from build123d import *

# Parameters (mm, degrees)
CROQUIS1_W              = 80
CROQUIS1_H              = 80
SALIENTE_EXTRUIR2_DEPTH = 2.7
CROQUIS2_R              = 2.5
CORTAR_EXTRUIR1_DEPTH   = 2.7
CROQUIS4_R              = 7.5
CORTAR_EXTRUIR2_DEPTH   = 2.7


with BuildPart() as part:
    # Croquis1 → Saliente-Extruir2 (new body)
    with BuildSketch(Plane.XY):
        with Locations((-42.7, 0)):
            Rectangle(CROQUIS1_W, CROQUIS1_H)
    extrude(amount=-SALIENTE_EXTRUIR2_DEPTH)

    # Croquis2 → Cortar-Extruir1 (cut)
    with BuildSketch(Plane(origin=(0, 0, -2.7), x_dir=(-1, 0, 0), z_dir=(0, 0, -1))):
        with Locations((67.7, 0)):
            Circle(CROQUIS2_R)
        with Locations((42.7, 0)):
            Circle(CROQUIS2_R)
    extrude(amount=-CORTAR_EXTRUIR1_DEPTH, mode=Mode.SUBTRACT)

    # Croquis4 → Cortar-Extruir2 (cut)
    with BuildSketch(Plane(origin=(0, 0, -2.7), x_dir=(-1, 0, 0), z_dir=(0, 0, -1))):
        with Locations((22.7, 23.2)):
            Circle(CROQUIS4_R)
    extrude(amount=-CORTAR_EXTRUIR2_DEPTH, mode=Mode.SUBTRACT)


solid = part.part
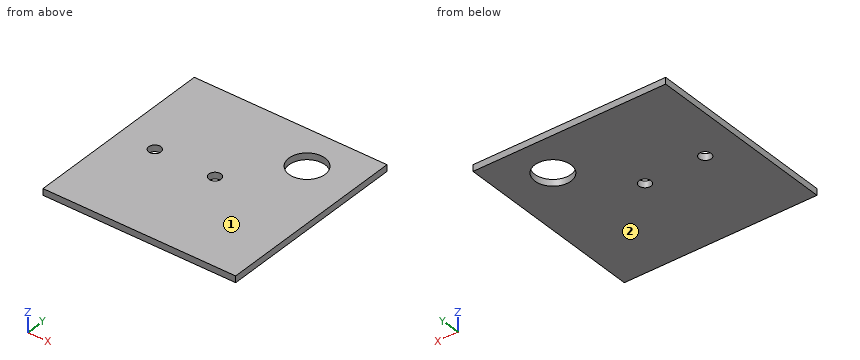
For this review, take the finished solid that the model builds, in its own axes (mm). Face numbers are marked on the shaded views. Coordinates: 2 decimals unless noted, no trailing zeros. Write each loop counter-clockwise with the first axis right and the second up, starting at its lowest first coordinate (ties: lowest second). Pieces come first, ordered by that corner, then holes. Notation, with made-up numbers: (18.5, 15.5) -> (67.5, 15.5) arc R15 ccw to (67.5, 25.5) -> close; hole circle Ø2 at (44, 46). An arc over 180 degrees is marked (long way). Write each question's results on one line, items separated by ' | '. Start each with the question number.
1) Wall thickness on L1, parallel to Y at x = -22.7, z = -2.05; L2, parallel to X at y = 1.5, z = -1.85; L3, parallel to Y at x = -67.7, z = -1.4: over which ranges is each line inside the solid? List them lowest first. Write a range as [from, to].
2) Consider section A-A (x = -67.7). Write out the cut boundary in (y, z), plus the area to 4 significant figures.
3) Consider section B-B (y = 23.2). Write out the cut boundary in (x, z), plus the area to 4 significant figures.
4) Consider section D-D (z = -2.05). Write out the cut boundary in (x, y), plus the area to 3 significant figures.
5) The part is to be moulded in two halves that separate along Z. For the marked faces 1 and 2, say which applies: +Z half, -Z half, draft (parallel to the pull), parting line (faces both ways), or undercut.
6) Consider section C-C (y = 0). Write out the cut boundary in (x, z).
Geometry says:
1) L1: [-40, 15.7], [30.7, 40] | L2: [-82.7, -69.7], [-65.7, -44.7], [-40.7, -2.7] | L3: [-40, -2.5], [2.5, 40]
2) outline: (-40, -2.7) -> (-2.5, -2.7) -> (-2.5, 0) -> (-40, 0) -> close; (2.5, -2.7) -> (40, -2.7) -> (40, 0) -> (2.5, 0) -> close | area: 202.5 mm^2
3) outline: (-82.7, -2.7) -> (-30.2, -2.7) -> (-30.2, 0) -> (-82.7, 0) -> close; (-15.2, -2.7) -> (-2.7, -2.7) -> (-2.7, 0) -> (-15.2, 0) -> close | area: 175.5 mm^2
4) outline: (-82.7, -40) -> (-2.7, -40) -> (-2.7, 40) -> (-82.7, 40) -> close; hole circle Ø5 at (-67.7, 0); hole circle Ø5 at (-42.7, 0); hole circle Ø15 at (-22.7, 23.2) | area: 6,180 mm^2
5) face 1: +Z half | face 2: -Z half
6) outline: (-82.7, -2.7) -> (-70.2, -2.7) -> (-70.2, 0) -> (-82.7, 0) -> close; (-65.2, -2.7) -> (-45.2, -2.7) -> (-45.2, 0) -> (-65.2, 0) -> close; (-40.2, -2.7) -> (-2.7, -2.7) -> (-2.7, 0) -> (-40.2, 0) -> close
